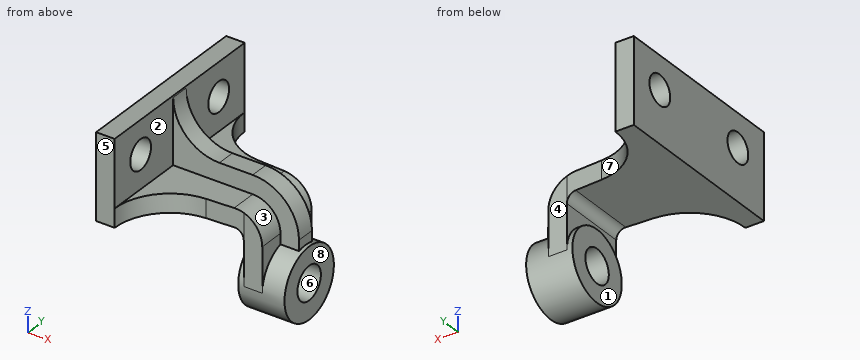
from build123d import *

# Parameters (mm, degrees)
F1_DEPTH    = 50
F2_DEPTH    = 19
F4_DEPTH    = 10
F5_R        = 5
F6_T1_DEPTH = 113
F7_R        = 8
F8_DEPTH    = 10
F11_W       = 28.4062897359
F11_H       = 10.0000000002
F12_DEPTH   = 5
F10_R       = 9
F13_DEPTH   = 25
F14_DEPTH   = 20


# Not quite as in the source:
# - a fillet or chamfer that OpenCascade refuses, or shapes differently, is made with other operations: its cross-section is extruded or revolved along the edge and cut away or added


with BuildPart() as f1:
    # F0 (on Front) → F1 (new body, symmetric)
    with BuildSketch(Plane.XZ):
        Polygon((0, 46), (0, 0), (58, 0), (58, 10), (10, 10), (10, 46), align=None)
    extrude(amount=F1_DEPTH, both=True)

    # F0 (on Front) → F2 (join, symmetric)
    with BuildSketch(Plane.XZ):
        Polygon((0, 46), (0, 0), (58, 0), (58, 10), (10, 10), (10, 46), align=None)
        Polygon((58, 10), (58, 0), (58, -29), (68, -29), (68, 10), align=None)
    extrude(amount=F2_DEPTH, both=True)

    # F3 (on face) → F4 (cut, through all)
    with BuildSketch(Plane.XY.offset(10)):
        with BuildLine():
            Line((58, -19), (38.4062897359, -20.0423617821))
            ThreePointArc((38.4062897359, -20.0423617821), (18.2306257793, -29.3579471457), (10, -50))
            Line((10, -50), (58, -50))
            Line((58, -50), (58, -19))
        make_face()
        with BuildLine():
            Line((58, 50), (10, 50))
            ThreePointArc((10, 50), (18.2306257793, 29.3579471457), (38.4062897359, 20.0423617821))
            Line((38.4062897359, 20.0423617821), (58, 19))
            Line((58, 19), (58, 50))
        make_face()
    extrude(amount=-F4_DEPTH, mode=Mode.SUBTRACT)

    # F5
    f5_edges = [f1.edges().sort_by_distance(p)[0] for p in [
        (58, 0, 0),
    ]]
    fillet(f5_edges, radius=F5_R)

    # F6: fillet of radius 15 on 1 edges, made by hand

    # F6_s2 → F6_t1 (cut)
    with BuildSketch(Plane.XZ.offset(-56.5)):
        with BuildLine():
            ThreePointArc((53, 10), (63.6066017178, 5.6066017178), (68, -5))
            Line((68, -5), (68, 10))
            Line((68, 10), (53, 10))
        make_face()
    extrude(amount=F6_T1_DEPTH, mode=Mode.SUBTRACT)

    # F7 (on face) → F8 (cut, through all)
    with BuildSketch(Plane.YZ.offset(10)):
        with Locations((-30, 28)):
            Circle(F7_R)
        with Locations((30, 28)):
            Circle(F7_R)
    extrude(amount=-F8_DEPTH, mode=Mode.SUBTRACT)

    # F11 (on Front) → F12 (join, symmetric)
    with BuildSketch(Plane.XZ):
        Polygon((10, 10), (10, 45.0000000683), (10, 46), (0, 46), (0, 0), (10, 0), align=None)
        with BuildLine():
            ThreePointArc((35, 20), (17.3223304462, 27.3223304945), (10, 45.0000000683))
            Line((10, 45.0000000683), (10, 10))
            Line((10, 10), (38.4062897359, 10))
            Line((38.4062897359, 10), (53, 10))
            ThreePointArc((53, 10), (55.5365296809, 9.7839783948), (58, 9.1421356237))
            ThreePointArc((58, 9.1421356237), (65.2474487139, 3.6602540378), (68, -5))
            Line((68, -5), (68, -29))
            Line((68, -29), (78, -29))
            Line((78, -29), (78, -5))
            ThreePointArc((78, -5), (70.6776695297, 12.6776695297), (53, 20))
            Line((53, 20), (35, 20))
        make_face()
        with Locations((24.2031448679, 4.9999999999)):
            Rectangle(F11_W, F11_H)
    extrude(amount=F12_DEPTH, both=True)

    # F10 (on offset) → F13 (join)
    with BuildSketch(Plane.YZ.offset(80)):
        with BuildLine():
            ThreePointArc((-19, -29), (0, -48), (19, -29))
            ThreePointArc((19, -29), (0, -10), (-19, -29))
        make_face()
        with Locations((0, -29)):
            Circle(F10_R, mode=Mode.SUBTRACT)
    extrude(amount=-F13_DEPTH)

    # F14 (cut, through all): faces of the model
    f14_faces = [f1.faces().sort_by_distance(p)[0] for p in [
        (78, 0, -24.7319215604),
        (68, -6.6350234662, -26.0867467093),
        (68, 6.6350234662, -26.0867467093),
    ]]
    extrude(f14_faces, amount=-F14_DEPTH, mode=Mode.SUBTRACT)


solid = f1.part
Build history of the part. All positions in model axes, mm. Face numbers are marked on the shaded views. A direction names the side the tool comes from. Round coordinates to 2 decimals unless told otherwise and drop trailing zeros. Write each loop counter-clockwise with the first axis right and the second up, starting at its lowest first coordinate (ties: lowest second). Pieces come first, ordered by that corner, then holes. Notation, with made-up numbers: (6.25, 52.5) - (49.25, 52.5) arc R24 ccw to (49.25, 78.5) - close; hole circle Ø2 at (60, 78.25). An arc over 180 degrees is marked (long way). One line per question, with ' | ' between items.
1. Drop flat-ended pins along their axis: pin 1 Ø8 at (x, z) = (65, -9.5) entering from -Y; pin 2 Ø6 at (x, y) = (68.5, -7.5) entering from -Z; pin 3 Ø1 at (y, z) = (-24.5, 5.5) entering from +X. Give the stop position or say it passes through.
Results are:
pin 1: y = -19 | pin 2: z = -47.46 | pin 3: x = 25.03
2. Mould opens along Y. For the marked faces 5, 6, 7 and 8 say: released by +Y, released by -Y, zero draft, split by the parting line, or undercut.
Results are:
face 5: released by -Y | face 6: undercut | face 7: released by +Y | face 8: zero draft
3. Band-saw the part on B-B, the plane z = -36.5. Write the cut outline in (x, y), and give its area (3 significant figures).
Results are:
outline: (55, -17.46) - (80, -17.46) - (80, -4.97) - (55, -4.97) - close; (55, 4.97) - (80, 4.97) - (80, 17.46) - (55, 17.46) - close | area: 624 mm^2
4. Drill centre lines: line 1 along Y through (x, z) = (4.5, 22); line 2 along Z through (x, y) = (4, -30); line 3 along Z through (x, y) = (15.5, -19.5). Where is each one in solid material? Low to high. Write a range as from..to.
Results are:
line 1: -50..-35.29, -24.71..24.71, 35.29..50 | line 2: 0..20, 36..46 | line 3: 0..10
5. Band-saw the part on C-C, the plane x = 14.5. Write the cut outline in (y, z), and give its area (3 significant figures).
Results are:
outline: (-34.2, 0) - (34.2, 0) - (34.2, 10) - (5, 10) - (5, 30.69) - (-5, 30.69) - (-5, 10) - (-34.2, 10) - close | area: 891 mm^2
6. Band-saw the part on A-A, the plane y = 0. Write the cut outline in (x, z).
Results are:
outline: (0, 0) - (53, 0) arc R5 cw to (58, -5) - (58, -10) - (55, -10) - (55, -20) - (80, -20) - (80, -10) - (78, -10) - (78, -5) arc R25 ccw to (53, 20) - (35, 20) arc R25 cw to (10, 45) - (10, 46) - (0, 46) - close; (55, -48) - (80, -48) - (80, -38) - (55, -38) - close
7. Tool access for the marked faces 1, 2, 3 and 4: list every direction of +Z, -Z, +X, -X, +Y, -Y with a clear straight run to the whole face (end or side of a thin tool).
Results are:
face 1: -Z, -X, +Y, -Y | face 2: +Z, +X | face 3: +Z, +X, -Y | face 4: +Z, -Z, +X, +Y
8. Band-saw the part on D-D, the plane z = 33.5. Write the cut outline in (x, y).
Results are:
outline: (0, -50) - (10, -50) - (10, -35.81) - (0, -35.81) - close; (0, -24.19) - (10, -24.19) - (10, -5) - (12.8, -5) - (12.8, 5) - (10, 5) - (10, 24.19) - (0, 24.19) - close; (0, 35.81) - (10, 35.81) - (10, 50) - (0, 50) - close
